Check sheet for the modelled part. Datum: model origin and axes. Units: mm. Give positions to 0.01 mm unless a question says otherwise; leave off trailing zeros. Loops run counter-clockwise (first coordinate to the right, second up) from the corner with the lowest first, then second, coordinate; pieces in that order, holes last.
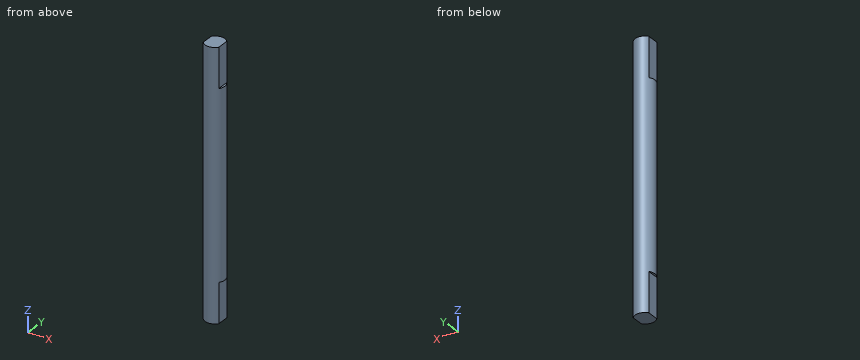
Autodesk Inventor part; units mm, degrees
ref_plane "YZ Plane" through (0, 0, 0) normal (1, 0, 0) x (0, 1, 0)
ref_plane "XZ Plane" through (0, 0, 0) normal (0, 1, 0) x (-1, 0, 0)
ref_plane "XY Plane" through (0, 0, 0) normal (0, 0, 1) x (1, 0, 0)
sketch "Sketch1" plane through (0, 0, 0) normal (0, 0, 1) x (1, 0, 0)
  circle A0 centre (0, 0) radius 6.35
  dimension "d0" = 12.7
extrude "Extrusion1" add sketch "Sketch1" along normal blind 170
sketch "Sketch2" plane through (0, 0, 170) normal (0, 0, 1) x (1, 0, 0)
  circle A0 centre (0, 0) radius 6.35
  line L0 (-5, 3.9144) -> (5, 3.9144) construction
  line L1 (-5, 3.9144) -> (5, 3.9144) construction
  line L2 (-5, -3.9144) -> (5, -3.9144) construction
  line L3 (-5, -3.9144) -> (5, -3.9144) construction
  circle A1 centre (0, 0) radius 6.35
  dimension "d3" = 10
  dimension "d4" = 0
  dimension "d5" = 10
  dimension "d6" = 0
thread "Thread1"
thread "Thread2"
sketch "Sketch3" plane through (0, 0, 170) normal (0, 0, 1) x (1, 0, 0)
  circle A0 centre (0, 0) radius 6.35
  line L0 (5.0019, 3.912) -> (5.0019, -3.912)
  arc A1 (5.0019, -3.912) -> (5.0019, 3.912) centre (0, 0) ccw
extrude "Extrusion2" cut sketch "Sketch3" against normal blind 25.4 contours A0 L0 picked at (5.2474, -0.9063)
sketch "Sketch4" plane through (0, 0, 170) normal (0, 0, 1) x (1, 0, 0)
  arc A0 (5.0019, 3.912) -> (5.0019, -3.912) centre (0, 0) ccw
  line L0 (-5.0019, 3.912) -> (-5.0019, -3.912)
  arc A1 (-5.0019, 3.912) -> (-5.0019, -3.912) centre (0, 0) ccw
extrude "Extrusion3" cut sketch "Sketch4" against normal blind 25.4
sketch "Sketch5" plane through (0, 0, 0) normal (0, 0, -1) x (-1, 0, 0)
  line L0 (-5.0019, -3.912) -> (-5.0019, 3.912)
  line L1 (-5.0019, 3.912) -> (-5.0019, -3.912)
  arc A0 (-5.0019, 3.912) -> (-5.0019, -3.912) centre (0, 0) ccw
extrude "Extrusion4" cut sketch "Sketch5" against normal blind 25.4
sketch "Sketch6" plane through (0, 0, 0) normal (0, 0, -1) x (-1, 0, 0)
  arc A0 (5.0019, -3.912) -> (5.0019, 3.912) centre (0, 0) ccw
  line L0 (5.0019, 3.912) -> (5.0019, -3.912)
  arc A1 (5.0019, -3.912) -> (5.0019, 3.912) centre (0, 0) ccw
extrude "Extrusion5" cut sketch "Sketch6" against normal blind 25.4
properties part number "Rear Axle2"
(1) Gauge pin test, flat ends, axial feed: pin 1 Ø1.5 at (x, z) = (3, 20.5) entering from +Y; pin 2 Ø5 at (x, y) = (-2.5, 0.5) entering from -Z; pin 3 Ø4 at (y, z) = (1.5, 13) entering from +X; pin 4 Ø1.1 at (x, y) = (6, -1) entering from -Z. Record the tip position at first contact, or that the pin passes through.
(2) Section check A-A on y = 0. Record the boundary of the cut face in (x, z), plus the area to 3 significant figures.
(3) Section check D-D on z = 55.5. Record the boundary of the cut face in (x, y).
(4) Material ranges on line 1 (X direction, y = 0.5, z = 62); line 2 (X direction, y = -3, z = 127); line 3 (Y direction, x = 2.25, z = 37), recorded low to high.
(5) Section check B-B on z = 12.5. Record the boundary of the cut face in (x, y).
(6) Section check C-C on x = 1.25. Record the boundary of the cut face in (y, z), plus the area to 3 significant figures.
Computed values:
1. pin 1: stops at y = 5.94
1. pin 2: stops at z = 0
1. pin 3: stops at x = 5
1. pin 4: stops at z = 25.4
2. outline: (-6.35, 25.4) - (-5, 25.4) - (-5, 0) - (5, 0) - (5, 25.4) - (6.35, 25.4) - (6.35, 144.6) - (5, 144.6) - (5, 170) - (-5, 170) - (-5, 144.6) - (-6.35, 144.6) - close
2. area: 2,020 mm2
3. outline: circle Ø12.7 at (0, 0)
4. line 1: x = -6.33 to 6.33
4. line 2: x = -5.6 to 5.6
4. line 3: y = -5.94 to 5.94
5. outline: (-5, -3.91) arc R6.35 ccw to (5, -3.91) - (5, 3.91) arc R6.35 ccw to (-5, 3.91) - close
6. outline: (-6.23, 0) - (6.23, 0) - (6.23, 170) - (-6.23, 170) - close
6. area: 2,120 mm2
